from build123d import *

# Parameters (mm, degrees)
SKETCH_1_W          = 20
SKETCH_1_H          = 31
EXTRUDE_1_DEPTH     = 3
SKETCH_3_R          = 3
SKETCH_3_R_2        = 1
EXTRUDE_2_DEPTH     = 3
SKETCH_4_R          = 1
CUT_EXTRUDE_1_DEPTH = 3
CHAMFER_1_SIZE      = 2


with BuildPart() as part:
    # Эскиз1 → Бобышка-Вытянуть1 (new body)
    with BuildSketch(Plane(origin=(0, 0, 0), x_dir=(1, 0, 0), z_dir=(0, 1, 0))):
        with Locations((-0.943604651, -8.91744186)):
            Rectangle(SKETCH_1_W, SKETCH_1_H)
    extrude(amount=EXTRUDE_1_DEPTH)

    # Эскиз3 → Бобышка-Вытянуть2 (add)
    with BuildSketch(Plane(origin=(0, 3, 0), x_dir=(1, 0, 0), z_dir=(0, 1, 0))):
        with Locations((-7.943604651, 0.58255814)):
            Circle(SKETCH_3_R)
        with Locations((-7.943604651, 0.58255814)):
            Circle(SKETCH_3_R_2, mode=Mode.SUBTRACT)
        with Locations((6.056395349, 0.58255814)):
            Circle(SKETCH_3_R)
        with Locations((6.056395349, 0.58255814)):
            Circle(SKETCH_3_R_2, mode=Mode.SUBTRACT)
        with Locations((-0.943604651, -18.41744186)):
            Circle(SKETCH_3_R)
        with Locations((-0.943604651, -18.41744186)):
            Circle(SKETCH_3_R_2, mode=Mode.SUBTRACT)
    extrude(amount=EXTRUDE_2_DEPTH)

    # Эскиз4 → Вырез-Вытянуть1 (cut)
    with BuildSketch(Plane(origin=(0, 3, 0), x_dir=(1, 0, 0), z_dir=(0, 1, 0))):
        with Locations((-0.943604651, -8.91744186)):
            Circle(SKETCH_4_R)
    extrude(amount=-CUT_EXTRUDE_1_DEPTH, mode=Mode.SUBTRACT)

    # Фаска1
    chamfer_1_edges = [part.edges().sort_by_distance(p)[0] for p in [
        (-1.943604651, 3, 8.91744186),
    ]]
    chamfer(chamfer_1_edges, length=CHAMFER_1_SIZE)


solid = part.part
Can you work these out from the model? Positions are in its coordinate system, mm. A direction names the side the tool comes from. Give positions to 0.01 mm unless a question says otherwise; leave off trailing zeros. Order: outer loops, then holes, each group sorted by start corner. A loop starts at its lowest first (then second) coordinate and runs counter-clockwise, first axis right, second up. Notation, with made-up numbers: M 72,49 L 98,49 A21 cw 98,73 Z; hole C 83,-36 d8. An arc over 180 degrees is marked long. Use one line per item in the form item = value.
Item 1: If I drill on line 1 along Y through (x, z) = (2.25, 14); line 2 along X through (y, z) = (2.9, 8); line 3 along Z through (x, y) = (-7.75, 4.15), over which ranges is the centre line in solid material (lowest first)? Write a range as [from, to].
Values follow:
line_1 = [0, 3]
line_2 = [-10.94, -3.69], [1.81, 9.06]
line_3 = [-3.58, -1.56], [0.4, 2.41]
Item 2: Will these pins go through, and if not, where does the flat tip stop? pin 1 Ø1 at (x, y) = (-2, 4.5) entering from +Z; pin 2 Ø4 at (x, z) = (-7, 10.5) entering from +Y; pin 3 Ø1.2 at (x, z) = (-0.94, 8.92) entering from -Y.
Values follow:
pin_1 = 21.37
pin_2 = 3
pin_3 = through
Item 3: For faces 5 (the flat face through (-1, 1, -6.583)), 6 (the cylindrical face through (-8.943, 4.479, -0.627)), which set-ups out of +Z, -Z, +X, -X, +Y, -Y let a thin tool reach every point of the face, with its end or its side?
Values follow:
face_5 = -Z, +X, -X, +Y, -Y
face_6 = +Y
Item 4: If we section it at D-D, the plane z = 17: Write out the boundary of the cut face in (x, y).
Values follow:
outline = M -10.94,0 L 9.06,0 L 9.06,3 L 1.7,3 L 1.7,6 L -3.59,6 L -3.59,3 L -10.94,3 Z
Item 5: Thinking about a two-plate mould opening in X: for faces 1 (the cylindrical face through (-5.08, 4.48, -1.48)), 2 (the flat face through (-6.7, 6, -0.6)), 3 (the flat face through (-10.944, 1, 9)), 4 (the flat face through (6, 3, -1)), which applies, pulls with the +X half, pulls with the -X half, needs draft (parallel to the pull), parting line crosses it, or undercut?
Values follow:
face_1 = undercut
face_2 = needs draft
face_3 = pulls with the -X half
face_4 = undercut
Item 6: If we section it at A-A, the plane y = 4.65: Write out the boundary of the cut face in (x, z).
Values follow:
outline = C -7.94,-0.58 d6; C -0.94,18.42 d6; C 6.06,-0.58 d6; hole C -7.94,-0.58 d2; hole C -0.94,18.42 d2; hole C 6.06,-0.58 d2
Item 7: If we section it at C-C, the plane x = -7.5: Write out the boundary of the cut face in (y, z).
Values follow:
outline = M 0,-6.58 L 3,-6.58 L 3,-3.55 L 6,-3.55 L 6,-1.48 L 3,-1.48 L 3,0.31 L 6,0.31 L 6,2.38 L 3,2.38 L 3,24.42 L 0,24.42 Z
Item 8: If we section it at B-B, the plane z = 2: Write out the boundary of the cut face in (x, y).
Values follow:
outline = M -10.94,0 L 9.06,0 L 9.06,3 L 7.58,3 L 7.58,6 L 4.53,6 L 4.53,3 L -6.42,3 L -6.42,6 L -9.47,6 L -9.47,3 L -10.94,3 Z
